Model file for the job. Use its own axes, mm. Give positions to 0.01 mm unless a question says otherwise; leave off trailing zeros. Loops run counter-clockwise (first coordinate to the right, second up) from the corner with the lowest first, then second, coordinate; pieces in that order, holes last. Notation, with made-up numbers: M 28,-1 L 55,-1 A17 cw 55,18 Z; hole C 56.5,-28 d11. An arc over 180 degrees is marked long. Answer in a Markdown table with one row per item.
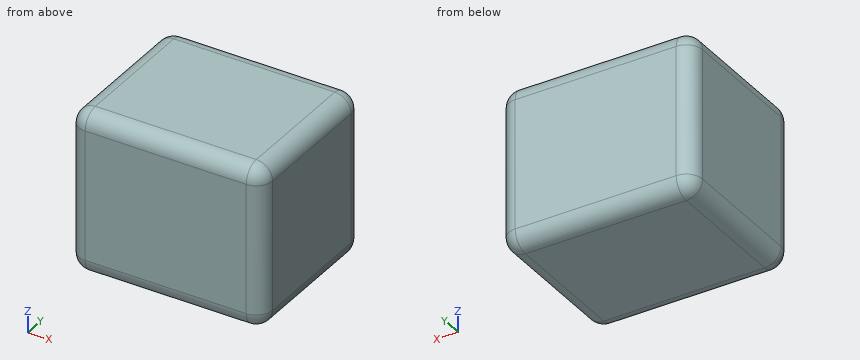
```python
from build123d import *

# Parameters (mm, degrees)
F0_W         = 60.5695545673
F0_H         = 49.7252251953
F1_DEPTH     = 50.8
F2_R         = 5.08
F3_R         = 5.08
F4_T1_DEPTH  = 40.64
F4_S5_W      = 5.08
F4_S5_H      = 5.08
F4_T6_DEPTH  = 5.08
F4_S11_W     = 5.08
F4_S11_H     = 5.08
F4_T12_DEPTH = 5.08
F4_S17_W     = 5.08
F4_S17_H     = 5.08
F4_T18_DEPTH = 5.08
F4_S23_W     = 5.08
F4_S23_H     = 5.08
F4_T24_DEPTH = 5.08
F4_S29_W     = 5.08
F4_S29_H     = 5.08
F4_T30_DEPTH = 5.08
F4_S35_W     = 5.08
F4_S35_H     = 5.08
F4_T36_DEPTH = 5.08
F4_S41_W     = 5.08
F4_S41_H     = 5.08
F4_T42_DEPTH = 5.08
F4_S47_W     = 5.08
F4_S47_H     = 5.08
F4_T48_DEPTH = 5.08


# Not quite as in the source:
# - a fillet or chamfer that OpenCascade refuses, or shapes differently, is made with other operations: its cross-section is extruded or revolved along the edge and cut away or added


with BuildPart() as f1:
    # F0 (on Top) → F1 (new body)
    with BuildSketch(Plane.XY):
        with Locations((3.8351900876, -0.2644965425)):
            Rectangle(F0_W, F0_H)
    extrude(amount=F1_DEPTH)

    # F2
    f2_edges = [f1.edges().sort_by_distance(p)[0] for p in [
        (3.83519, -25.127109, 50.8),
        (-26.449587, -0.264497, 50.8),
        (3.83519, 24.598116, 50.8),
        (34.119967, -0.264497, 50.8),
    ]]
    fillet(f2_edges, radius=F2_R)

    # F3
    f3_edges = [f1.edges().sort_by_distance(p)[0] for p in [
        (3.83519, -25.127109, 0),
        (34.119967, -0.264497, 0),
        (3.83519, 24.598116, 0),
        (-26.449587, -0.264497, 0),
    ]]
    fillet(f3_edges, radius=F3_R)

    # F4: fillet of radius 5.08 on 4 edges, made by hand

    # F4_s2 → F4_t1 (cut)
    with BuildSketch(Plane.XY.offset(5.08)):
        with BuildLine():
            ThreePointArc((-21.3695871961, 24.5981160551), (-24.9616896445, 23.1102185036), (-26.4495871961, 19.5181160551))
            Line((-26.4495871961, 19.5181160551), (-26.4495871961, 24.5981160551))
            Line((-26.4495871961, 24.5981160551), (-21.3695871961, 24.5981160551))
        make_face()
        with BuildLine():
            ThreePointArc((-26.4495871961, -20.0471091402), (-24.9616896445, -23.6392115886), (-21.3695871961, -25.1271091402))
            Line((-21.3695871961, -25.1271091402), (-26.4495871961, -25.1271091402))
            Line((-26.4495871961, -25.1271091402), (-26.4495871961, -20.0471091402))
        make_face()
        with BuildLine():
            ThreePointArc((29.0399673712, 24.5981160551), (32.6320698197, 23.1102185036), (34.1199673712, 19.5181160551))
            Line((34.1199673712, 19.5181160551), (34.1199673712, 24.5981160551))
            Line((34.1199673712, 24.5981160551), (29.0399673712, 24.5981160551))
        make_face()
        with BuildLine():
            ThreePointArc((34.1199673712, -20.0471091402), (32.6320698197, -23.6392115886), (29.0399673712, -25.1271091402))
            Line((29.0399673712, -25.1271091402), (34.1199673712, -25.1271091402))
            Line((34.1199673712, -25.1271091402), (34.1199673712, -20.0471091402))
        make_face()
    extrude(amount=F4_T1_DEPTH, mode=Mode.SUBTRACT)


with BuildPart() as f4_tool4:
    # F4_s5 → F4_t6 (new body)
    with BuildSketch(Plane.YZ.offset(29.0399673712)):
        with Locations((-22.5871091402, 2.54)):
            Rectangle(F4_S5_W, F4_S5_H)
    extrude(amount=F4_T6_DEPTH)

    # F4_s7 → F4_t8 (revolve, cut)
    with BuildSketch(Plane(origin=(29.0399673712, -20.0471091402, 5.08), x_dir=(0, 0.7071067812, 0.7071067812), z_dir=(0, 0.7071067812, -0.7071067812))):
        with BuildLine():
            ThreePointArc((0, -5.08), (5.08, 0), (0, 5.08))
            Line((0, 5.08), (0, -5.08))
        make_face()
    revolve(axis=Axis((29.0399673712, -20.0471091402, 5.08), (1, 0, 0)), mode=Mode.SUBTRACT)


with BuildPart() as f1_1:
    add(f1.part)

    # F4_t3: cut F4_tool4
    add(f4_tool4.part, mode=Mode.SUBTRACT)


with BuildPart() as f4_tool10:
    # F4_s11 → F4_t12 (new body)
    with BuildSketch(Plane.YZ.offset(29.0399673712)):
        with Locations((-22.5871091402, 48.26)):
            Rectangle(F4_S11_W, F4_S11_H)
    extrude(amount=F4_T12_DEPTH)

    # F4_s13 → F4_t14 (revolve, cut)
    with BuildSketch(Plane(origin=(29.0399673712, -20.0471091402, 45.72), x_dir=(0, 0.7071067812, -0.7071067812), z_dir=(0, -0.7071067812, -0.7071067812))):
        with BuildLine():
            ThreePointArc((0, -5.08), (5.08, 0), (0, 5.08))
            Line((0, 5.08), (0, -5.08))
        make_face()
    revolve(axis=Axis((29.0399673712, -20.0471091402, 45.72), (1, 0, 0)), mode=Mode.SUBTRACT)


with BuildPart() as f1_2:
    add(f1_1.part)

    # F4_t9: cut F4_tool10
    add(f4_tool10.part, mode=Mode.SUBTRACT)


with BuildPart() as f4_tool16:
    # F4_s17 → F4_t18 (new body)
    with BuildSketch(Plane.XZ.offset(-19.5181160551)):
        with Locations((31.5799673712, 2.54)):
            Rectangle(F4_S17_W, F4_S17_H)
    extrude(amount=-F4_T18_DEPTH)

    # F4_s19 → F4_t20 (revolve, cut)
    with BuildSketch(Plane(origin=(29.0399673712, 19.5181160551, 5.08), x_dir=(-0.7071067812, 0, 0.7071067812), z_dir=(-0.7071067812, 0, -0.7071067812))):
        with BuildLine():
            ThreePointArc((0, -5.08), (5.08, 0), (0, 5.08))
            Line((0, 5.08), (0, -5.08))
        make_face()
    revolve(axis=Axis((29.0399673712, 19.5181160551, 5.08), (0, 1, 0)), mode=Mode.SUBTRACT)


with BuildPart() as f1_3:
    add(f1_2.part)

    # F4_t15: cut F4_tool16
    add(f4_tool16.part, mode=Mode.SUBTRACT)


with BuildPart() as f4_tool22:
    # F4_s23 → F4_t24 (new body)
    with BuildSketch(Plane.XZ.offset(-19.5181160551)):
        with Locations((31.5799673712, 48.26)):
            Rectangle(F4_S23_W, F4_S23_H)
    extrude(amount=-F4_T24_DEPTH)

    # F4_s25 → F4_t26 (revolve, cut)
    with BuildSketch(Plane(origin=(29.0399673712, 19.5181160551, 45.72), x_dir=(-0.7071067812, 0, -0.7071067812), z_dir=(0.7071067812, 0, -0.7071067812))):
        with BuildLine():
            ThreePointArc((0, -5.08), (5.08, 0), (0, 5.08))
            Line((0, 5.08), (0, -5.08))
        make_face()
    revolve(axis=Axis((29.0399673712, 19.5181160551, 45.72), (0, 1, 0)), mode=Mode.SUBTRACT)


with BuildPart() as f1_4:
    add(f1_3.part)

    # F4_t21: cut F4_tool22
    add(f4_tool22.part, mode=Mode.SUBTRACT)


with BuildPart() as f4_tool28:
    # F4_s29 → F4_t30 (new body)
    with BuildSketch(Plane.YZ.offset(-21.3695871961)):
        with Locations((-22.5871091402, 2.54)):
            Rectangle(F4_S29_W, F4_S29_H)
    extrude(amount=-F4_T30_DEPTH)

    # F4_s31 → F4_t32 (revolve, cut)
    with BuildSketch(Plane(origin=(-21.3695871961, -20.0471091402, 5.08), x_dir=(0, 0.7071067812, 0.7071067812), z_dir=(0, -0.7071067812, 0.7071067812))):
        with BuildLine():
            ThreePointArc((0, -5.08), (5.08, 0), (0, 5.08))
            Line((0, 5.08), (0, -5.08))
        make_face()
    revolve(axis=Axis((-21.3695871961, -20.0471091402, 5.08), (-1, 0, 0)), mode=Mode.SUBTRACT)


with BuildPart() as f1_5:
    add(f1_4.part)

    # F4_t27: cut F4_tool28
    add(f4_tool28.part, mode=Mode.SUBTRACT)


with BuildPart() as f4_tool34:
    # F4_s35 → F4_t36 (new body)
    with BuildSketch(Plane.YZ.offset(-21.3695871961)):
        with Locations((-22.5871091402, 48.26)):
            Rectangle(F4_S35_W, F4_S35_H)
    extrude(amount=-F4_T36_DEPTH)

    # F4_s37 → F4_t38 (revolve, cut)
    with BuildSketch(Plane(origin=(-21.3695871961, -20.0471091402, 45.72), x_dir=(0, 0.7071067812, -0.7071067812), z_dir=(0, 0.7071067812, 0.7071067812))):
        with BuildLine():
            ThreePointArc((0, -5.08), (5.08, 0), (0, 5.08))
            Line((0, 5.08), (0, -5.08))
        make_face()
    revolve(axis=Axis((-21.3695871961, -20.0471091402, 45.72), (-1, 0, 0)), mode=Mode.SUBTRACT)


with BuildPart() as f1_6:
    add(f1_5.part)

    # F4_t33: cut F4_tool34
    add(f4_tool34.part, mode=Mode.SUBTRACT)


with BuildPart() as f4_tool40:
    # F4_s41 → F4_t42 (new body)
    with BuildSketch(Plane.XZ.offset(-19.5181160551)):
        with Locations((-23.9095871961, 2.54)):
            Rectangle(F4_S41_W, F4_S41_H)
    extrude(amount=-F4_T42_DEPTH)

    # F4_s43 → F4_t44 (revolve, cut)
    with BuildSketch(Plane(origin=(-21.3695871961, 19.5181160551, 5.08), x_dir=(0.7071067812, 0, 0.7071067812), z_dir=(-0.7071067812, 0, 0.7071067812))):
        with BuildLine():
            ThreePointArc((0, -5.08), (5.08, 0), (0, 5.08))
            Line((0, 5.08), (0, -5.08))
        make_face()
    revolve(axis=Axis((-21.3695871961, 19.5181160551, 5.08), (0, 1, 0)), mode=Mode.SUBTRACT)


with BuildPart() as f1_7:
    add(f1_6.part)

    # F4_t39: cut F4_tool40
    add(f4_tool40.part, mode=Mode.SUBTRACT)


with BuildPart() as f4_tool46:
    # F4_s47 → F4_t48 (new body)
    with BuildSketch(Plane.XZ.offset(-19.5181160551)):
        with Locations((-23.9095871961, 48.26)):
            Rectangle(F4_S47_W, F4_S47_H)
    extrude(amount=-F4_T48_DEPTH)

    # F4_s49 → F4_t50 (revolve, cut)
    with BuildSketch(Plane(origin=(-21.3695871961, 19.5181160551, 45.72), x_dir=(0.7071067812, 0, -0.7071067812), z_dir=(0.7071067812, 0, 0.7071067812))):
        with BuildLine():
            ThreePointArc((0, -5.08), (5.08, 0), (0, 5.08))
            Line((0, 5.08), (0, -5.08))
        make_face()
    revolve(axis=Axis((-21.3695871961, 19.5181160551, 45.72), (0, 1, 0)), mode=Mode.SUBTRACT)


with BuildPart() as f1_8:
    add(f1_7.part)

    # F4_t45: cut F4_tool46
    add(f4_tool46.part, mode=Mode.SUBTRACT)


solid = f1_8.part
```
(1) Wall check: L1, parallel to X at y = 13, z = 46; L2, parallel to Y at x = 30.5, z = 16.5; L3, parallel to Y at x = 28, z = 5. Give the ranges that are in metal, low to high.
Established:
| item | result |
|---|---|
| L1 | x = -26.44 to 34.11 |
| L2 | y = -24.91 to 24.38 |
| L3 | y = -25.13 to 24.6 |
(2) Saw through at A-A, the plane y = 21. Give the cut face in (x, z).
Established:
| item | result |
|---|---|
| outline | M -26.23,5.08 A4.86 ccw -21.37,0.22 L 29.04,0.22 A4.86 ccw 33.9,5.08 L 33.9,45.72 A4.86 ccw 29.04,50.58 L -21.37,50.58 A4.86 ccw -26.23,45.72 Z |
(3) Saw through at B-B, the plane z = 4. Give the cut face in (x, y).
Established:
| item | result |
|---|---|
| outline | M -26.33,-20.05 A4.96 ccw -21.37,-25.01 L 29.04,-25.01 A4.96 ccw 34,-20.05 L 34,19.52 A4.96 ccw 29.04,24.48 L -21.37,24.48 A4.96 ccw -26.33,19.52 Z |
